Build history of the part. All positions in model axes, mm. A direction names the side the tool comes from. Give positions to 0.01 mm unless a question says otherwise; leave off trailing zeros. Write each loop counter-clockwise with the first axis right and the second up, starting at its lowest first coordinate (ties: lowest second). Pieces come first, ordered by that corner, then holes. Notation, with made-up numbers: M 56.5,65 L 93.5,65 A3 cw 93.5,69 Z; hole C -8.75,-4.75 d11. An arc over 180 degrees is marked long. One line per item, written item: value. Start each with the question number.
from build123d import *

# Parameters (mm, degrees)
SKETCH1_R           = 57.5
BOSS_EXTRUDE1_DEPTH = 1328
SKETCH3_R           = 82.5
BOSS_EXTRUDE2_DEPTH = 150
CUT_EXTRUDE1_DEPTH  = 150
CIRPATTERN1_COUNT   = 12


with BuildPart() as part:
    # Sketch1 → Boss-Extrude1 (new body)
    with BuildSketch(Plane.XY):
        Circle(SKETCH1_R)
    extrude(amount=BOSS_EXTRUDE1_DEPTH)

    # Sketch3 → Boss-Extrude2 (add)
    with BuildSketch(Plane(origin=(0, 0, 0), x_dir=(-1, 0, 0), z_dir=(0, 0, -1))):
        Circle(SKETCH3_R)
    extrude(amount=BOSS_EXTRUDE2_DEPTH)

    # Sketch5 → Cut-Extrude1 (cut)
    with BuildSketch(Plane(origin=(0, 0, -150), x_dir=(-1, 0, 0), z_dir=(0, 0, -1))):
        with BuildLine():
            Line((-13.805552215, 81.336687467), (-5.048873049, 57.277909188))
            ThreePointArc((-5.048873049, 57.277909188), (0, 57.5), (5.048873049, 57.277909188))
            Line((5.048873049, 57.277909188), (13.805552215, 81.336687467))
            ThreePointArc((13.805552215, 81.336687467), (0, 82.5), (-13.805552215, 81.336687467))
        make_face()
    cut_extrude1 = extrude(amount=-CUT_EXTRUDE1_DEPTH, mode=Mode.SUBTRACT)

    # CirPattern1: Cut-Extrude1 ×12 about axis
    cirpattern1_axis = Axis((0, 0, 0), (0, 0, 1))
    for i in range(1, CIRPATTERN1_COUNT):
        add(cut_extrude1.rotate(cirpattern1_axis, i * 360 / CIRPATTERN1_COUNT), mode=Mode.SUBTRACT)


solid = part.part
1) Mould opens along Y. For faces 4 (the face through (-26.46, -64.56, -76.05)), 5 (the face through (-1, 1, 1328)), 6 (the face through (9.49, 69.48, -76.05)) say: released by +Y, released by -Y, zero draft, split by the parting line, or undercut.
2) Drop flat-ended pins along their axis: P1, Ø12, axis at x = 11.5, y = -67, coming from the +Z side; P2, Ø6, axis at y = 38.5, z = 589.5, coming from the -X side; P3, Ø3, axis at y = 8.5, z = 564.5, coming from the -X side; P4, Ø4, axis at x = 4.5, y = -63, coming from the +Z side. Give the stop position or say it passes through.
3) Band-saw the part on A-A (z = 776.5). List the corners of the cut face in (x, y).
4) Tool access for faces 1 (the face through (64.91, 26.52, -76.05)), 2 (the face through (-17, -67, 0)), 3 (the face through (9.366, -69.139, -76.05)): list every direction of +Z, -Z, +X, -X, +Y, -Y with a clear straight run to the whole face (end or side of a thin tool).
5) Probe line 1 along Z through (x, y) = (50.5, 47.5); line 2 along X through (y, z) = (53, -71); line 3 along X through (y, z) = (-39, -29.5). List the from-to ranges inside material, lowest first. Write a range as from..to.
Model answer:
1. face 4: undercut
1. face 5: zero draft
1. face 6: released by +Y
2. P1: stops at z = 0
2. P2: stops at x = -45.23
2. P3: stops at x = -57.07
2. P4: passes through
3. outline: C 0,0 d115
4. face 1: +Z, -Z
4. face 2: +Z, -X, -Y
4. face 3: +Z, -Z, -Y
5. line 1: z = -150..0
5. line 2: x = -63.22..-40.07, -24.42..24.42, 40.07..63.22
5. line 3: x = -52.1..52.1
